Autodesk Inventor part; units mm, degrees
ref_plane "YZ Plane" through (0, 0, 0) normal (1, 0, 0) x (0, 1, 0)
ref_plane "XZ Plane" through (0, 0, 0) normal (0, 1, 0) x (-1, 0, 0)
ref_plane "XY Plane" through (0, 0, 0) normal (0, 0, 1) x (1, 0, 0)
sketch "Sketch1" plane through (0, 0, 0) normal (0, 1, 0) x (-1, 0, 0)
  line L0 (10.07, 20.05) -> (-10.07, 20.05)
  line L1 (-10.07, 20.05) -> (-10.07, -20.05)
  line L2 (-10.07, -20.05) -> (10.07, -20.05)
  line L3 (10.07, -20.05) -> (10.07, 20.05)
  point P0 (0, 0)
  dimension "d0" = 40.1
  dimension "d1" = 20.14
  dimension "d2" = 10.07
  dimension "d3" = 20.05
extrude "Plate1" add sketch "Sketch1" along normal blind 1.5
sketch "Sketch2" plane through (10.07, 0, 21.55) normal (0, 0, -1) x (-1, 0, 0)
  line L0 (20.14, 0) -> (0, 0)
  line L1 (0, 0) -> (0, 45.48)
  line L2 (0, 45.48) -> (20.14, 45.48)
  line L3 (20.14, 45.48) -> (20.14, 0)
edge flange "Flange1" height 45.48 angle 90 thickness 1.5 bend radius 0.31 thickness toward (0, 0, -1) relief tear relief width 1.5 relief depth 0.75 corner gap 0.31 corner form 0 edges at (0, 1.5, 20.05) (0, 1.5, -20.05) wall of the first edge with corners at (-10.07, 0, 21.55) (10.07, 0, 21.55) (10.07, 45.48, 21.55) (-10.07, 45.48, 21.55)
bend "Bend1"
corner "Corner1"
sketch "Sketch3" plane through (10.07, 45.48, -21.55) normal (0, 0, -1) x (-1, 0, 0)
  circle A0 centre (17.595, -1.24) radius 0.7835
  circle A1 centre (2.545, -1.24) radius 0.7835
  circle A2 centre (2.545, -16.34) radius 0.7835
  circle A3 centre (17.595, -16.34) radius 0.7835
  point P0 (10.07, -45.48)
hole "Hole1" at (7.525, 44.24, -21.55) at (-7.525, 44.24, -21.55) at (-7.525, 29.14, -21.55) at (7.525, 29.14, -21.55) direction (0, 0, 1) diameter 2.1 depth 1.5
sketch "Sketch4" plane through (-10.07, 45.48, 21.55) normal (0, 0, 1) x (1, 0, 0)
  circle A0 centre (2.545, -1.24) radius 0.7835
  circle A1 centre (17.595, -1.24) radius 0.7835
  circle A2 centre (3.07, -8.86) radius 0.7835
  circle A3 centre (17.07, -8.86) radius 0.7835
  point P0 (10.07, -45.48)
sketch "Sketch5" plane through (-10.07, 45.48, 21.55) normal (0, 0, 1) x (1, 0, 0)
  circle A0 centre (10.07, -16.16) radius 0.7835
  point P0 (10.07, -45.48)
hole "Hole2" at (-7.525, 44.24, 21.55) at (7.525, 44.24, 21.55) at (-7, 36.62, 21.55) at (7, 36.62, 21.55) direction (0, 0, -1) diameter 2.1 depth 1.5
hole "Hole3" at (0, 29.32, 21.55) direction (0, 0, -1) diameter 2.1 depth 1.5
sketch "Sketch6" plane through (0, 0, 0) normal (0, -1, 0) x (1, 0, 0)
  circle A0 centre (7.0007, -3.08) radius 1.55
  circle A1 centre (7, -17.08) radius 1.55
  circle A2 centre (-7, -17.08) radius 1.55
  circle A3 centre (-7, -3.08) radius 1.55
  point P0 (0, 0)
extrude "Cut1" cut sketch "Sketch6" against normal blind 1.5
equation "\"d20\" = Thickness"
equation "\"d27\" = Thickness"
equation "\"d34\" = Thickness"
equation "\"d36\" = Thickness"
equation "\"d4\" = Thickness"
equation "\"d5\" = BendReliefWidth"
equation "\"d6\" = BendReliefDepth"
equation "\"d7\" = MinimumRemnant"
equation "\"d8\" = TransitionRadius"
equation "\"d11\" = BendRadius"
equation "\"d12\" = CornerReliefSize"
equation "\"d13\" = GapSize"
equation "\"d14\" = JacobiRadiusSize"
equation "\"BendReliefWidth\" = Thickness"
equation "\"BendReliefDepth\" = 0.5 * Thickness"
equation "\"CornerReliefSize\" = 4 * Thickness"
equation "\"MinimumRemnant\" = 2 * Thickness"
equation "\"TransitionRadius\" = BendRadius"
equation "\"JacobiRadiusSize\" = BendRadius"
equation "\"GapSize\" = Thickness"
properties part number "axis_25_top_frame" material "Aluminum 6061-AHC"
Input: part model. Units: mm. Frame: model coordinates. A direction names the side the tool comes from. Give positions to 0.01 mm unless a question says otherwise; leave off trailing zeros. Order: outer loops, then holes, each group sorted by start corner. A loop starts at its lowest first (then second) coordinate and runs counter-clockwise, first axis right, second up. Notation, with made-up numbers: M 79,24.5 L 88,24.5 A22 cw 88,34.5 Z; hole C 75.25,10 d8. An arc over 180 degrees is marked long. Return JSON: item names as keys, results as strings.
Item 1: First-contact query: P1, Ø1.5, axis at x = 2, z = 11, coming from the +Y side; P2, Ø1.3, axis at x = 7.525, y = 29.14, coming from the -Z side. Flat tips, straight axial feed; report the tip coordinate or a pass-through.
Solutions:
{"P1": "y = 1.5", "P2": "z = 20.05"}
Item 2: Ray query, probe 1 along X at (y, z) = (36.62, 20.6); probe 2 along Z at (x, y) = (-1, 11.5); probe 3 along X at (y, z) = (29.14, -21.1) (3 decimals). Return the intervals inside material, ascending.
Solutions:
{"probe 1": "-10.07 to -8.05, -5.95 to 5.95, 8.05 to 10.07", "probe 2": "-21.55 to -20.05, 20.05 to 21.55", "probe 3": "-10.07 to -8.575, -6.475 to 6.475, 8.575 to 10.07"}
Item 3: Access query for faces 5 (the cylindrical face through (7.21, 43.24, 20.79)), 6 (the cylindrical face through (-0.32, 28.32, 20.79)), 7 (the cylindrical face through (-8.41, 29.704, -20.79)). Directions: +Z, -Z, +X, -X, +Y, -Y. A direction counts if a zero-diameter tool reaches every point of the face in a straight line with its end or side. Return the directions, or none.
Solutions:
{"face 5": "+Z, -Z", "face 6": "+Z", "face 7": "-Z"}
Item 4: Cut plane D-D (y = 5). Return loops of the section in (x, z), then the cut area to 3 significant figures.
Solutions:
{"outline": "M -10.07,-21.55 L 10.07,-21.55 L 10.07,-20.05 L -10.07,-20.05 Z; M -10.07,20.05 L 10.07,20.05 L 10.07,21.55 L -10.07,21.55 Z", "area": "60.4 mm^2"}
Item 5: Pull-direction query (Z, two-part tool) for faces 1 (the cylindrical face through (7.21, 45.24, -20.79)), 2 (the flat face through (0, 24, -21.55)), 3 (the flat face through (0, 23, -20.05)), 4 (the cylindrical face through (5.86, 0.74, -2.03)); classes: +Z half, -Z half, draft (parallel to the pull), parting line (faces both ways), or undercut.
Solutions:
{"face 1": "draft", "face 2": "-Z half", "face 3": "undercut", "face 4": "undercut"}
Item 6: Cut plane A-A (z = -17.08). Return loops of the section in (x, y), then the cut area to 3 significant figures.
Solutions:
{"outline": "M -10.07,0 L -8.55,0 L -8.55,1.5 L -10.07,1.5 Z; M -5.45,0 L 5.45,0 L 5.45,1.5 L -5.45,1.5 Z; M 8.55,0 L 10.07,0 L 10.07,1.5 L 8.55,1.5 Z", "area": "20.9 mm^2"}
Item 7: Cut plane B-B (y = 36.62). Return loops of the section in (x, z), then the cut area to 3 significant figures.
Solutions:
{"outline": "M -10.07,-21.55 L 10.07,-21.55 L 10.07,-20.05 L -10.07,-20.05 Z; M -10.07,20.05 L -8.05,20.05 L -8.05,21.55 L -10.07,21.55 Z; M -5.95,20.05 L 5.95,20.05 L 5.95,21.55 L -5.95,21.55 Z; M 8.05,20.05 L 10.07,20.05 L 10.07,21.55 L 8.05,21.55 Z", "area": "54.1 mm^2"}
Item 8: Cut plane C-C (x = 0). Return loops of the section in (y, z), then the cut area to 3 significant figures.
Solutions:
{"outline": "M 0,-19.74 A1.81 ccw 1.81,-21.55 L 45.48,-21.55 L 45.48,-20.05 L 1.81,-20.05 A0.31 cw 1.5,-19.74 L 1.5,19.74 A0.31 cw 1.81,20.05 L 28.27,20.05 L 28.27,21.55 L 1.81,21.55 A1.81 ccw 0,19.74 Z; M 30.37,20.05 L 45.48,20.05 L 45.48,21.55 L 30.37,21.55 Z", "area": "192 mm^2"}
